The model under review builds one solid part; all positions refer to its coordinate system, in mm. Face numbers are marked on the shaded views. A direction names the side the tool comes from. Coordinates: 2 decimals unless noted, no trailing zeros. Order: outer loops, then holes, each group sorted by start corner. A loop starts at its lowest first (then second) coordinate and runs counter-clockwise, first axis right, second up. Notation, with made-up numbers: M 33,58.5 L 65,58.5 A32 ccw 65,86.5 Z; hole C 44,36 d9. An arc over 180 degrees is marked long. One line per item, written item: value.
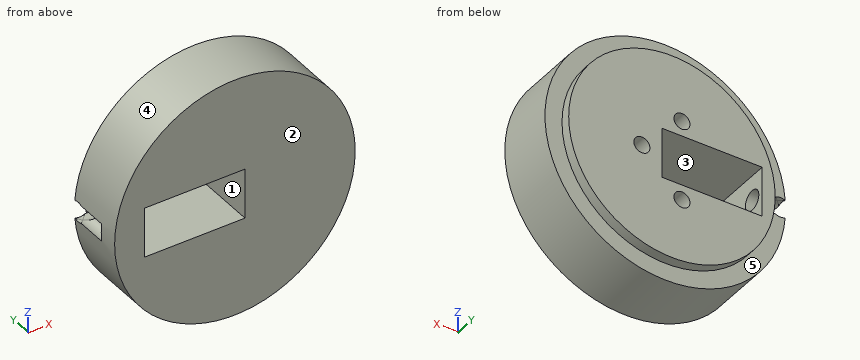
```python
from build123d import *

# Parameters (mm, degrees)
CYLINDER014005814004009_R           = 1
CYLINDER014005814004009_DEPTH       = 12
CYLINDER014005814004009_PITCH_ANGLE = 90
CYLINDER014005814004010_R           = 1
CYLINDER014005814004010_DEPTH       = 4
CYLINDER014005814004010_ROLL_ANGLE  = 90
CYLINDER014005814004011_R           = 0.8
CYLINDER014005814004011_DEPTH       = 4
CYLINDER014005814004011_ROLL_ANGLE  = 90
CYLINDER014005814004012_R           = 0.8
CYLINDER014005814004012_DEPTH       = 4
CYLINDER014005814004012_ROLL_ANGLE  = 90
CYLINDER014005814004013_R           = 0.8
CYLINDER014005814004013_DEPTH       = 4
CYLINDER014005814004013_ROLL_ANGLE  = 90
BOX209_W                            = 10
BOX209_H                            = 11
BOX209_DEPTH                        = 5
CYLINDER014005814004008_R           = 10.3
CYLINDER014005814004008_DEPTH       = 7
CYLINDER014005814004008_ROLL_ANGLE  = 90
CYLINDER014005814004007_R           = 12
CYLINDER014005814004007_DEPTH       = 6
CYLINDER014005814004007_ROLL_ANGLE  = 90
CUT061098127_PLACEMENT_ANGLE        = 180


with BuildPart() as obj1:
    # Cylinder014005814004009 → Cylinder014005814004009 (new body)
    with BuildSketch(Plane.XY):
        Circle(CYLINDER014005814004009_R)
    extrude(amount=CYLINDER014005814004009_DEPTH)


with BuildPart() as obj1_1:
    # Cylinder014005814004009 pitch: moved
    add(obj1.part.rotate(Axis((0, 0, 0), (0, 1, 0)), CYLINDER014005814004009_PITCH_ANGLE))


with BuildPart() as obj1_2:
    # Cylinder014005814004009 placement: moved
    add(obj1_1.part.moved(Location((0, -5.5, 0))))


with BuildPart() as obj2:
    # Cylinder014005814004010 → Cylinder014005814004010 (new body)
    with BuildSketch(Plane.XY):
        Circle(CYLINDER014005814004010_R)
    extrude(amount=CYLINDER014005814004010_DEPTH)


with BuildPart() as obj2_1:
    # Cylinder014005814004010 roll: moved
    add(obj2.part.rotate(Axis((0, 0, 0), (1, 0, 0)), CYLINDER014005814004010_ROLL_ANGLE))


with BuildPart() as obj2_2:
    # Cylinder014005814004010 placement: moved
    add(obj2_1.part.moved(Location((11.5, -2, 0))))


with BuildPart() as obj3:
    # Cylinder014005814004011 → Cylinder014005814004011 (new body)
    with BuildSketch(Plane.XY):
        Circle(CYLINDER014005814004011_R)
    extrude(amount=CYLINDER014005814004011_DEPTH)


with BuildPart() as obj3_1:
    # Cylinder014005814004011 roll: moved
    add(obj3.part.rotate(Axis((0, 0, 0), (1, 0, 0)), CYLINDER014005814004011_ROLL_ANGLE))


with BuildPart() as obj3_2:
    # Cylinder014005814004011 placement: moved
    add(obj3_1.part.moved(Location((-3, -3, 0))))


with BuildPart() as obj4:
    # Cylinder014005814004012 → Cylinder014005814004012 (new body)
    with BuildSketch(Plane.XY):
        Circle(CYLINDER014005814004012_R)
    extrude(amount=CYLINDER014005814004012_DEPTH)


with BuildPart() as obj4_1:
    # Cylinder014005814004012 roll: moved
    add(obj4.part.rotate(Axis((0, 0, 0), (1, 0, 0)), CYLINDER014005814004012_ROLL_ANGLE))


with BuildPart() as obj4_2:
    # Cylinder014005814004012 placement: moved
    add(obj4_1.part.moved(Location((1, -3, 4))))


with BuildPart() as obj5:
    # Cylinder014005814004013 → Cylinder014005814004013 (new body)
    with BuildSketch(Plane.XY):
        Circle(CYLINDER014005814004013_R)
    extrude(amount=CYLINDER014005814004013_DEPTH)


with BuildPart() as obj5_1:
    # Cylinder014005814004013 roll: moved
    add(obj5.part.rotate(Axis((0, 0, 0), (1, 0, 0)), CYLINDER014005814004013_ROLL_ANGLE))


with BuildPart() as obj5_2:
    # Cylinder014005814004013 placement: moved
    add(obj5_1.part.moved(Location((1, -3, -4))))


with BuildPart() as fusion001089087:
    # Box209 → Box209 (new body)
    with BuildSketch(Plane(origin=(-1, -7, -2.5), x_dir=(1, 0, 0), z_dir=(0, 0, 1))):
        with Locations((5, 5.5)):
            Rectangle(BOX209_W, BOX209_H)
    extrude(amount=BOX209_DEPTH)

    # Fusion001089087: union obj1, obj2, obj3, obj4, obj5
    add(obj1_2.part)
    add(obj2_2.part)
    add(obj3_2.part)
    add(obj4_2.part)
    add(obj5_2.part)


with BuildPart() as bat005:
    # Cylinder014005814004008 → Cylinder014005814004008 (new body)
    with BuildSketch(Plane.XY):
        Circle(CYLINDER014005814004008_R)
    extrude(amount=CYLINDER014005814004008_DEPTH)


with BuildPart() as bat005_1:
    # Cylinder014005814004008 roll: moved
    add(bat005.part.rotate(Axis((0, 0, 0), (1, 0, 0)), CYLINDER014005814004008_ROLL_ANGLE))


with BuildPart() as bat005_2:
    # Cylinder014005814004008 placement: moved
    add(bat005_1.part)


with BuildPart() as obj6:
    # Cylinder014005814004007 → Cylinder014005814004007 (new body)
    with BuildSketch(Plane.XY):
        Circle(CYLINDER014005814004007_R)
    extrude(amount=CYLINDER014005814004007_DEPTH)


with BuildPart() as obj6_1:
    # Cylinder014005814004007 roll: moved
    add(obj6.part.rotate(Axis((0, 0, 0), (1, 0, 0)), CYLINDER014005814004007_ROLL_ANGLE))


with BuildPart() as obj6_2:
    # Cylinder014005814004007 placement: moved
    add(obj6_1.part)

    # Fusion001089086: union bat005
    add(bat005_2.part)

    # Cut061098127: cut Fusion001089087
    add(fusion001089087.part, mode=Mode.SUBTRACT)


with BuildPart() as obj6_3:
    # Cut061098127 placement: moved
    add(obj6_2.part.moved(Location((0, -28, 37))).rotate(Axis((0, -28, 37), (0, 0, 1)), CUT061098127_PLACEMENT_ANGLE))


solid = obj6_3.part
```
(1) Tool access review of the marked faces 1 and 2: name each direction out of +Z, -Z, +X, -X, +Y, -Y from which nothing blocks a thin tool from reaching the whole face with its end or side.
Geometry results:
face 1: +Y, -Y
face 2: +Z, -Z, +X, -X, -Y
(2) We need section B-B, the plane x = -4.5. State the section outline as (y, z) points, plus the area to 3 significant figures.
Geometry results:
outline: M -28,25.88 L -22,25.88 L -22,27.74 L -21,27.74 L -21,34.5 L -28,34.5 Z; M -28,39.5 L -21,39.5 L -21,46.26 L -22,46.26 L -22,48.12 L -28,48.12 Z
area: 117 mm2
(3) Insertion check: pin 1 Ø1 at (y, z) = (-27, 36.5) entering from +X; pin 2 Ø1.8 at (y, z) = (-22.5, 37) entering from -X; pin 3 Ø1.5 at (y, z) = (-22, 45) entering from -X; pin 4 Ø1.3 at (x, z) = (3, 37) entering from +Y. Each pin has a flat end and moves straight along its axis. Give the tip position at first contact, or say it passes through.
Geometry results:
pin 1: stops at x = 12
pin 2: stops at x = 1
pin 3: stops at x = -9.56
pin 4: stops at y = -25
(4) For L1, parallel to Z at x = -0.75, y = -24.75; L2, parallel to Z at x = -6, y = -26.25; L3, parallel to Z at x = -10.75, y = -24, list the stretches that pass through material, from the lowest coordinate up.
Geometry results:
L1: z = 25.02 to 32.24, 33.76 to 34.5, 39.5 to 40.24, 41.76 to 48.98
L2: z = 26.61 to 34.5, 39.5 to 47.39
L3: z = 31.67 to 36.34, 37.66 to 42.33
(5) We need section D-D, the plane z = 30.25. State the section outline as (x, y) points.
Geometry results:
outline: M -9.92,-28 L 9.92,-28 L 9.92,-22 L 7.78,-22 L 7.78,-21 L -7.78,-21 L -7.78,-22 L -9.92,-22 Z
(6) We need section C-C, the plane y = -26.5. State the section outline as (x, z) points.
Geometry results:
outline: C 0,37 d24; hole M -9,34.5 L 1,34.5 L 1,39.5 L -9,39.5 Z
(7) Mouldability with a two-part tool opening along X and no side actions: class the marked faces 3, 4 and 5 as +X half, -X half, draft (parallel to the pull), parting line (faces both ways), or undercut.
Geometry results:
face 3: undercut
face 4: parting line
face 5: draft
(8) We need section A-A, the plane y = -24.5. State the section outline as (x, z) points.
Geometry results:
outline: M -11.97,36.12 A12 ccw long -11.97,37.88 A1 cw long Z; hole M -9,34.5 L 1,34.5 L 1,39.5 L -9,39.5 Z; hole C -1,33 d1.6; hole C -1,41 d1.6; hole C 3,37 d1.6
